Read the model definition and answer for the solid it produces. Units are mm, in the model's axes. A direction names the side the tool comes from. Give positions to 0.01 mm unless a question says otherwise; leave off trailing zeros. Order: outer loops, then holes, each group sorted by start corner. A loop starts at its lowest first (then second) coordinate and runs counter-clockwise, first axis right, second up. Notation, with made-up numbers: (78.25, 75) - (108.25, 75) arc R28 cw to (108.25, 111) - close; hole circle Ø5 at (54.25, -24.75). An arc over 180 degrees is marked (long way). Answer as CSV lines item,"result". Start each with the question number.
from build123d import *

# Parameters (mm, degrees)
F1_DEPTH = 1117.6
F2_DEPTH = 304.8
F4_DEPTH = 406.4


with BuildPart() as f1:
    # F0 (on Front) → F1 (new body)
    with BuildSketch(Plane.XZ):
        with BuildLine():
            ThreePointArc((502.252486, 76.2), (385.798311, 330.490035), (152.4, 484.601114))
            ThreePointArc((152.4, 484.601114), (0, 508), (-152.4, 484.601114))
            ThreePointArc((-152.4, 484.601114), (-385.798311, 330.490035), (-502.252486, 76.2))
            Line((-502.252486, 76.2), (-160.643705, 76.2))
            ThreePointArc((-160.643705, 76.2), (0, 177.8), (160.643705, 76.2))
            Line((160.643705, 76.2), (502.252486, 76.2))
        make_face()
        with BuildLine():
            Line((-160.643705, 76.2), (-502.252486, 76.2))
            ThreePointArc((-502.252486, 76.2), (-508, 0), (-502.252486, -76.2))
            Line((-502.252486, -76.2), (-160.643705, -76.2))
            ThreePointArc((-160.643705, -76.2), (-177.8, 0), (-160.643705, 76.2))
        make_face()
        with BuildLine():
            ThreePointArc((177.8, 0), (173.457907, 39.05374), (160.643705, 76.2))
            ThreePointArc((160.643705, 76.2), (0, 177.8), (-160.643705, 76.2))
            ThreePointArc((-160.643705, 76.2), (-177.8, 0), (-160.643705, -76.2))
            ThreePointArc((-160.643705, -76.2), (0, -177.8), (160.643705, -76.2))
            ThreePointArc((160.643705, -76.2), (173.457907, -39.05374), (177.8, 0))
        make_face()
        with BuildLine():
            ThreePointArc((508, 0), (506.561084, 38.208225), (502.252486, 76.2))
            Line((502.252486, 76.2), (160.643705, 76.2))
            ThreePointArc((160.643705, 76.2), (173.457907, 39.05374), (177.8, 0))
            ThreePointArc((177.8, 0), (173.457907, -39.05374), (160.643705, -76.2))
            Line((160.643705, -76.2), (502.252486, -76.2))
            ThreePointArc((502.252486, -76.2), (506.561084, -38.208225), (508, 0))
        make_face()
        with BuildLine():
            ThreePointArc((-152.4, -484.601114), (0, -508), (152.4, -484.601114))
            ThreePointArc((152.4, -484.601114), (385.798311, -330.490035), (502.252486, -76.2))
            Line((502.252486, -76.2), (160.643705, -76.2))
            ThreePointArc((160.643705, -76.2), (0, -177.8), (-160.643705, -76.2))
            Line((-160.643705, -76.2), (-502.252486, -76.2))
            ThreePointArc((-502.252486, -76.2), (-385.798311, -330.490035), (-152.4, -484.601114))
        make_face()
    extrude(amount=F1_DEPTH)

    # F0 (on Front) → F2 (join)
    with BuildSketch(Plane.XZ):
        with BuildLine():
            Line((-152.4, 484.601114), (-152.4, 772.510841))
            ThreePointArc((-152.4, 772.510841), (-787.4, 0), (-152.4, -772.510841))
            Line((-152.4, -772.510841), (-152.4, -484.601114))
            ThreePointArc((-152.4, -484.601114), (-385.798311, -330.490035), (-502.252486, -76.2))
            ThreePointArc((-502.252486, -76.2), (-508, 0), (-502.252486, 76.2))
            ThreePointArc((-502.252486, 76.2), (-385.798311, 330.490035), (-152.4, 484.601114))
        make_face()
        with BuildLine():
            ThreePointArc((152.4, -772.510841), (608.275645, -499.9995), (787.4, 0))
            ThreePointArc((787.4, 0), (608.275645, 499.9995), (152.4, 772.510841))
            Line((152.4, 772.510841), (152.4, 484.601114))
            ThreePointArc((152.4, 484.601114), (385.798311, 330.490035), (502.252486, 76.2))
            ThreePointArc((502.252486, 76.2), (506.561084, 38.208225), (508, 0))
            ThreePointArc((508, 0), (506.561084, -38.208225), (502.252486, -76.2))
            ThreePointArc((502.252486, -76.2), (385.798311, -330.490035), (152.4, -484.601114))
            Line((152.4, -484.601114), (152.4, -772.510841))
        make_face()
    extrude(amount=F2_DEPTH)

    # F3 (on face) → F4 (cut)
    with BuildSketch(Plane.XZ.offset(1117.6)):
        with BuildLine():
            ThreePointArc((-160.643705, -76.2), (-177.8, 0), (-160.643705, 76.2))
            Line((-160.643705, 76.2), (-502.252486, 76.2))
            ThreePointArc((-502.252486, 76.2), (-508, 0), (-502.252486, -76.2))
            Line((-502.252486, -76.2), (-160.643705, -76.2))
        make_face()
        with BuildLine():
            ThreePointArc((160.643705, -76.2), (173.457907, -39.05374), (177.8, 0))
            ThreePointArc((177.8, 0), (173.457907, 39.05374), (160.643705, 76.2))
            ThreePointArc((160.643705, 76.2), (0, 177.8), (-160.643705, 76.2))
            ThreePointArc((-160.643705, 76.2), (-177.8, 0), (-160.643705, -76.2))
            ThreePointArc((-160.643705, -76.2), (0, -177.8), (160.643705, -76.2))
        make_face()
        with BuildLine():
            ThreePointArc((160.643705, 76.2), (173.457907, 39.05374), (177.8, 0))
            ThreePointArc((177.8, 0), (173.457907, -39.05374), (160.643705, -76.2))
            Line((160.643705, -76.2), (502.252486, -76.2))
            ThreePointArc((502.252486, -76.2), (506.561084, -38.208225), (508, 0))
            ThreePointArc((508, 0), (506.561084, 38.208225), (502.252486, 76.2))
            Line((502.252486, 76.2), (160.643705, 76.2))
        make_face()
    extrude(amount=-F4_DEPTH, mode=Mode.SUBTRACT)


solid = f1.part
(1) Section A-A, the plane y = -812.5 is taken. Write down the section's boundary in (x, z).
(2) Section C-C, the plane z = 617.5 is taken. Write down the section's boundary in (x, y), and give its area (3 significant figures).
(3) Determine the mould class of faces 1 (the flat face through (-334, -917, -76.2)), 2 (the flat face through (-7, -1117.6, -289)), 3 (the cylindrical face through (-787.254, -150.266, 15.168)) for opening direction Z: released by +Z, released by -Z, zero draft, split by the parting line, or undercut.
(4) Straight lines are drawn through the part: line 1 (Y direction, x = -677, z = 210.5); line 2 (Y direction, x = -122, z = -4.5); line 3 (Z direction, x = -77, y = -669). For each, find the intervals that lie inside material, in ascending order. Write a range as [from, to].
(5) Which of the six approach directions +Z, -Z, +X, -X, +Y, -Y give full straight-line access (tool end or side, diameter ignored) to faces 4 (the cylindrical face through (-508, -505, 1)), 5 (the cylindrical face through (2.807, -917.245, 177.778)), 6 (the flat face through (-152.4, -150, -631)), 7 (the flat face through (334, -917, 76.2)), 8 (the flat face through (152.4, -150, 631))?
(6) Section B-B, the plane y = -607 is taken. Write down the section's boundary in (x, z), and give its area (3 significant figures).
(7) Section D-D, the plane x = 124.5 is taken. Write down the section's boundary in (y, z), and give its area (3 significant figures).
(8) Flat-ended cylindrical pins translate along their axes: pin 1 Ø6 at (x, z) = (-118.5, -399) entering from +Y; pin 2 Ø1.5 at (x, y) = (303.5, -800.5) entering from +Z; pin 3 Ø2 at (y, z) = (-561, 194) entering from -X; pin 4 Ø10 at (y, z) = (-447.5, -167.5) entering from +X. Find the tip coordinate at first contact, or state that the pin passes through.
Checks:
1,outline,"(-502.25, -76.2) arc R508 ccw to (-152.4, -484.6) arc R508 ccw to (152.4, -484.6) arc R508 ccw to (502.25, -76.2) - (160.64, -76.2) arc R177.8 cw to (-160.64, -76.2) - close; (-502.25, 76.2) - (-160.64, 76.2) arc R177.8 cw to (160.64, 76.2) - (502.25, 76.2) arc R508 ccw to (152.4, 484.6) arc R508 ccw to (-152.4, 484.6) arc R508 ccw to start"
2,outline,"(-488.56, -304.8) - (-152.4, -304.8) - (-152.4, 0) - (-488.56, 0) - close; (152.4, -304.8) - (488.56, -304.8) - (488.56, 0) - (152.4, 0) - close"
2,area,"205,000 mm²"
3,face 1,"undercut"
3,face 2,"zero draft"
3,face 3,"split by the parting line"
4,line 1,"y = [-304.8, 0]"
4,line 2,"y = [-711.2, 0]"
4,line 3,"z = [-502.13, 502.13]"
5,face 4,"-X, -Y"
5,face 5,"-Y"
5,face 6,"-Z, +Y, -Y"
5,face 7,"+X, -X, -Y"
5,face 8,"+Z, +Y, -Y"
6,outline,"(-502.25, -76.2) arc R508 ccw to (-152.4, -484.6) arc R508 ccw to (152.4, -484.6) arc R508 ccw to (502.25, -76.2) arc R508 ccw to (508, 0) arc R508 ccw to (502.25, 76.2) arc R508 ccw to (152.4, 484.6) arc R508 ccw to (-152.4, 484.6) arc R508 ccw to (-502.25, 76.2) arc R508 ccw to start"
6,area,"811,000 mm²"
7,outline,"(-1117.6, -492.51) - (0, -492.51) - (0, 492.51) - (-1117.6, 492.51) - (-1117.6, 126.94) - (-711.2, 126.94) - (-711.2, -126.94) - (-1117.6, -126.94) - close"
7,area,"998,000 mm²"
8,pin 1,"stops at y = 0"
8,pin 2,"stops at z = 407.93"
8,pin 3,"stops at x = -469.91"
8,pin 4,"stops at x = 481.31"
